```python
from build123d import *

# Parameters (mm, degrees)
PAD_DEPTH    = 15
FILLET_R     = 7
FILLET001_R  = 1
SKETCH001_R  = 1.5
POCKET_DEPTH = 32.001


with BuildPart() as part:
    # Sketch → Pad (new body)
    with BuildSketch(Plane.XY):
        Polygon((-26, 0), (0, 0), (0, 12), (6, 12), (6, 0), (26, 0), (26, -3), (-26, -3), align=None)
    extrude(amount=PAD_DEPTH)

    # Fillet
    fillet_edges = [part.edges().sort_by_distance(p)[0] for p in [
        (3, 12, 0),
        (3, 12, 15),
    ]]
    fillet(fillet_edges, radius=FILLET_R)

    # Fillet001
    fillet001_edges = [part.edges().sort_by_distance(p)[0] for p in [
        (26, -1.5, 0),
        (26, -1.5, 15),
        (-26, -1.5, 0),
        (-26, -1.5, 15),
    ]]
    fillet(fillet001_edges, radius=FILLET001_R)

    # Sketch001 (on Face8 of Fillet001) → Pocket (cut, through all)
    with BuildSketch(Plane.YZ.offset(6)):
        with Locations((8, 7.5)):
            Circle(SKETCH001_R)
    extrude(amount=-POCKET_DEPTH, mode=Mode.SUBTRACT)


solid = part.part
```
Work out the finished part from the listing and answer in its coordinate system (mm). A direction names the side the tool comes from. Round coordinates to 2 decimals unless told otherwise and drop trailing zeros. Order: outer loops, then holes, each group sorted by start corner. A loop starts at its lowest first (then second) coordinate and runs counter-clockwise, first axis right, second up.
Q1. A cutting plane is placed at D-D, the plane z = 5.5. Determine the outline of the cut face in (x, y), then the cut area to 3 significant figures.
Solution:
outline: (-26, -3) - (26, -3) - (26, 0) - (6, 0) - (6, 11.84) - (0, 11.84) - (0, 0) - (-26, 0) - close
area: 227 mm2
Q2. A cutting plane is placed at B-B, the plane y = 8. Determine the outline of the cut face in (x, z), then the cut area to 3 significant figures.
Solution:
outline: (0, 0.68) - (6, 0.68) - (6, 6) - (0, 6) - close; (0, 9) - (6, 9) - (6, 14.32) - (0, 14.32) - close
area: 63.9 mm2
Q3. Given pin 1 Ø3.5 at (y, z) = (8, 8.5) entering from +X; pin 2 Ø3.5 at (y, z) = (8, 7.5) entering from -X; pin 3 Ø5 at (x, y) = (-3, 6) entering from +Z; pin 4 Ø7.5 at (x, z) = (-10, 6) entering from +Y, each flat-ended and moving along its own axis, determine where each tip first touches the part or whether it passes through.
Solution:
pin 1: stops at x = 6
pin 2: stops at x = 0
pin 3: passes through
pin 4: stops at y = 0
Q4. A tool of negligible diameter and unlimited length cuts with its end or side. For faces 4 (the flat face through (16, 0, 7)), 5 (the flat face through (0, -1, 0)), 6 (the flat face through (-13, 0, 7)), from which of +Z, -Z, +X, -X, +Y, -Y can it reach the whole face along a straight path? Write none if from no direction.
Solution:
face 4: +Z, -Z, +X, +Y
face 5: -Z, +X, -X, +Y, -Y
face 6: +Z, -Z, -X, +Y
Q5. A cutting plane is placed at C-C, the plane x = -12.5. Determine the outline of the cut face in (y, z).
Solution:
outline: (-3, 0) - (0, 0) - (0, 15) - (-3, 15) - close
Q6. The mould has two halves that part along Z. Classify faces 1 (the cylindrical face through (-25.699, -1.479, 0.285)), 2 (the flat face through (0, 6, 7)), 3 (the cylindrical face through (3, 6.8, 6.6)): pulls with the +Z half, pulls with the -Z half, needs draft (parallel to the pull), parting line crosses it, or undercut.
Solution:
face 1: pulls with the -Z half
face 2: needs draft
face 3: undercut
Q7. A cutting plane is placed at A-A, the plane z = 7.5. Determine the outline of the cut face in (x, y), then the cut area to 3 significant figures.
Solution:
outline: (-26, -3) - (26, -3) - (26, 0) - (6, 0) - (6, 6.5) - (0, 6.5) - (0, 0) - (-26, 0) - close; (0, 9.5) - (6, 9.5) - (6, 12) - (0, 12) - close
area: 210 mm2
Q8. Find the intervals of material crossed by line 1 along X through (y, z) = (5.5, 4); line 2 along Y through (x, z) = (-4.5, 0.5); line 3 along Z through (x, y) = (4, 8), in increasing order.
Solution:
line 1: x = 0 to 6
line 2: y = -3 to 0
line 3: z = 0.68 to 6, 9 to 14.32
